from build123d import *

# Parameters (mm, degrees)
SKETCH001_W     = 14.830339
SKETCH001_H     = 37.894496
SKETCH001_W_2   = 11.332046
SKETCH001_H_2   = 38.12416
POCKET_DEPTH    = 7.401
SKETCH002_R     = 0.825
POCKET001_DEPTH = 7.401
POCKET002_DEPTH = 1


with BuildPart() as part:
    # Sketch → Revolution (revolve)
    with BuildSketch(Plane.XZ):
        Polygon((0, 0), (4.5, 0), (4.5, 3.5), (1.5, 3.5), (1.5, 4), (4, 4), (4, 5), (15, 5), (15, 7.4), (1.5, 7.4), (1.5, 8.7), (10, 8.7), (10, 20.2), (6, 20.2), (6, 21.2), (2, 21.2), (2, 22.9), (1.5, 22.9), (1.5, 26.2), (0, 26.2), align=None)
    revolve(axis=Axis((0, 0, 0), (0, 0, 1)))

    # Sketch001 (on Face9 of Revolution) → Pocket (cut, through all)
    with BuildSketch(Plane(origin=(0, 0, 7.4), x_dir=(-1, 0, 0), z_dir=(0, 0, 1))):
        with Locations((-17.415169, -0.751627)):
            Rectangle(SKETCH001_W, SKETCH001_H)
        with Locations((15.666023, -0.866459)):
            Rectangle(SKETCH001_W_2, SKETCH001_H_2)
    extrude(amount=-POCKET_DEPTH, mode=Mode.SUBTRACT)

    # Sketch002 (on Face12 of Pocket) → Pocket001 (cut, through all)
    with BuildSketch(Plane(origin=(0, 0, 7.4), x_dir=(-1, 0, 0), z_dir=(0, 0, 1))):
        with Locations((-7.5, 10.75)):
            Circle(SKETCH002_R)
        with Locations((7.5, 10.75)):
            Circle(SKETCH002_R)
        with Locations((7.5, -10.75)):
            Circle(SKETCH002_R)
        with Locations((-7.5, -10.75)):
            Circle(SKETCH002_R)
        with BuildLine():
            ThreePointArc((1.9, 17.255435), (0, 19.155435), (-1.9, 17.255435))
            Line((-1.9, 17.255435), (-1.9, 12.65))
            ThreePointArc((-1.9, 12.65), (0, 10.75), (1.9, 12.65))
            Line((1.9, 12.65), (1.9, 17.255435))
        make_face()
        with BuildLine():
            ThreePointArc((-1.9, -16.247692), (0, -18.147692), (1.9, -16.247692))
            Line((1.9, -16.247692), (1.9, -12.65))
            ThreePointArc((1.9, -12.65), (0, -10.75), (-1.9, -12.65))
            Line((-1.9, -12.65), (-1.9, -16.247692))
        make_face()
    extrude(amount=-POCKET001_DEPTH, mode=Mode.SUBTRACT)

    # Sketch003 (on Face7 of Pocket001) → Pocket002 (cut)
    with BuildSketch(Plane(origin=(0, 0, 5), x_dir=(1, 0, 0), z_dir=(0, 0, -1))):
        with BuildLine():
            ThreePointArc((-5.75, 14.896887), (-7.5, 16.646887), (-9.25, 14.896887))
            Line((-9.25, 14.896887), (-9.25, 10.75))
            ThreePointArc((-9.25, 10.75), (-7.5, 9), (-5.75, 10.75))
            Line((-5.75, 10.75), (-5.75, 14.896887))
        make_face()
        with BuildLine():
            ThreePointArc((9.25, 14.479509), (7.5, 16.229509), (5.75, 14.479509))
            Line((5.75, 14.479509), (5.75, 10.75))
            ThreePointArc((5.75, 10.75), (7.5, 9), (9.25, 10.75))
            Line((9.25, 10.75), (9.25, 14.479509))
        make_face()
        with BuildLine():
            ThreePointArc((5.75, -14.269869), (7.5, -16.019869), (9.25, -14.269869))
            Line((9.25, -14.269869), (9.25, -10.75))
            ThreePointArc((9.25, -10.75), (7.5, -9), (5.75, -10.75))
            Line((5.75, -10.75), (5.75, -14.269869))
        make_face()
        with BuildLine():
            ThreePointArc((-9.25, -14.048632), (-7.5, -15.798632), (-5.75, -14.048632))
            Line((-5.75, -14.048632), (-5.75, -10.75))
            ThreePointArc((-5.75, -10.75), (-7.5, -9), (-9.25, -10.75))
            Line((-9.25, -10.75), (-9.25, -14.048632))
        make_face()
    extrude(amount=-POCKET002_DEPTH, mode=Mode.SUBTRACT)


solid = part.part
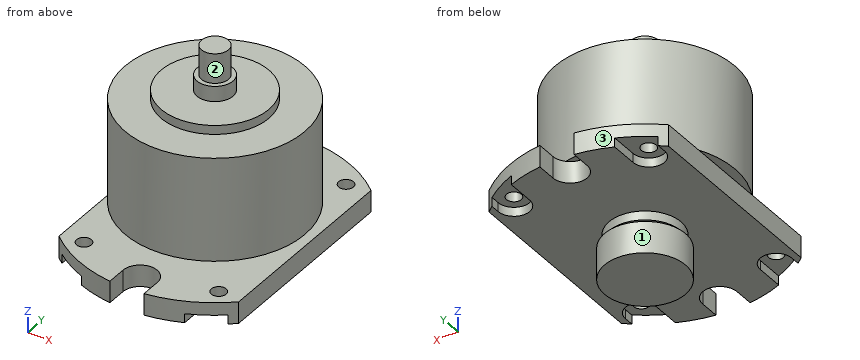
Work out the finished part from the listing and answer in its coordinate system (mm). Face numbers are marked on the shaded views. A direction names the side the tool comes from. Round coordinates to 2 decimals unless told otherwise and drop trailing zeros. Order: outer loops, then holes, each group sorted by start corner. A loop starts at its lowest first (then second) coordinate and runs counter-clockwise, first axis right, second up. Notation, with made-up numbers: M 89.5,61 L 111.5,61 A14 cw 111.5,68 Z; hole C 13.5,75.5 d11. An arc over 180 degrees is marked long. One line per item, written item: value.
Q1. Find section A-A on x = 7.5. Write down the section's boundary in (y, z) (3 decimals).
Derived:
outline: M -12.99,6 L -11.575,6 L -11.575,7.4 L -12.99,7.4 Z; M -9.925,6 L -9,6 L -9,5 L 9,5 L 9,6 L 9.925,6 L 9.925,7.4 L -9.925,7.4 Z; M -6.614,8.7 L 6.614,8.7 L 6.614,20.2 L -6.614,20.2 Z; M 11.575,6 L 12.99,6 L 12.99,7.4 L 11.575,7.4 Z
Q2. Find section B-B on x = 3.5. Write down the section's boundary in (y, z).
Derived:
outline: M -14.59,5 L -1.94,5 L -1.94,4 L 1.94,4 L 1.94,5 L 14.59,5 L 14.59,7.4 L -14.59,7.4 Z; M -9.37,8.7 L 9.37,8.7 L 9.37,20.2 L 4.87,20.2 L 4.87,21.2 L -4.87,21.2 L -4.87,20.2 L -9.37,20.2 Z; M -2.83,0 L 2.83,0 L 2.83,3.5 L -2.83,3.5 Z
Q3. For the marked faces 1, 2 and 3, determine the directions among +Z, -Z, +X, -X, +Y, -Y from which every point of the face is accessible in a straight line to the end or side of a thin tool.
Derived:
face 1: -Z
face 2: +Z
face 3: +Z, -Z, -X, +Y
Q4. Straight lines are drawn through the part: line 1 (Z direction, x = 0, y = -3.5); line 2 (Z direction, x = -6.25, y = -6); line 3 (Z direction, x = 5.25, y = -0.75). For each, find the intervals that lie inside material, in ascending order.
Derived:
line 1: 0 to 3.5, 4 to 7.4, 8.7 to 21.2
line 2: 5 to 7.4, 8.7 to 20.2
line 3: 5 to 7.4, 8.7 to 21.2
Q5. Flat-ended cylindrical pins translate along their axes: pin 1 (4 mm diameter, centred on x = -4, y = -9, fed in from +Z); pin 2 (4 mm diameter, centred on x = 1, z = 16, fed in from +Y); pin 3 (5 mm diameter, centred on x = 3.5, z = 12.5, fed in from -Y); pin 4 (1.3 mm diameter, centred on x = 7.5, y = 10.75, fed in from -Z). Find the tip coordinate at first contact, or state that the pin passes through.
Derived:
pin 1: z = 20.2
pin 2: y = 10
pin 3: y = -9.95
pin 4: through
Q6. Find section D-D on z = 2. Write down the section's boundary in (x, y), then the cut area to 3 significant figures.
Derived:
outline: C 0,0 d9
area: 63.6 mm²
Q7. Find section C-C on x = -5. Write down the section's boundary in (y, z), then the cut area to 3 significant figures.
Derived:
outline: M -14.14,5 L 14.14,5 L 14.14,7.4 L -14.14,7.4 Z; M -8.66,8.7 L 8.66,8.7 L 8.66,20.2 L 3.32,20.2 L 3.32,21.2 L -3.32,21.2 L -3.32,20.2 L -8.66,20.2 Z
area: 274 mm²
